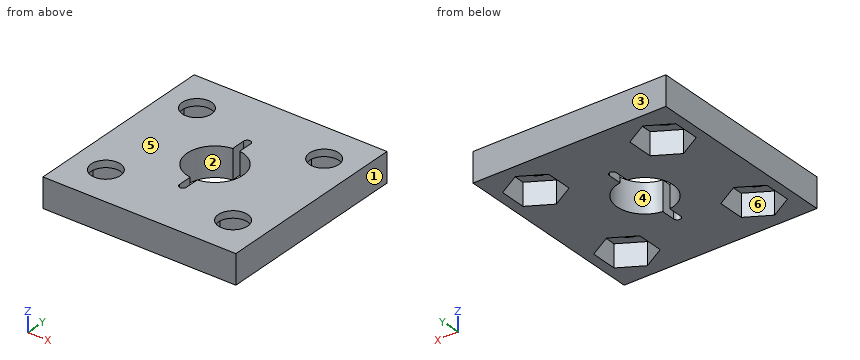
from build123d import *

# Parameters (mm, degrees)
SKETCH1_W           = 35.052
SKETCH1_H           = 35.814
SKETCH1_R           = 2.667
BOSS_EXTRUDE1_DEPTH = 5.334
CUT_EXTRUDE1_DEPTH  = 4.064
SKETCH3_R           = 5.08
CUT_EXTRUDE2_DEPTH  = 6.334
CUT_EXTRUDE3_DEPTH  = 6.334


with BuildPart() as part:
    # Sketch1 → Boss-Extrude1 (new body)
    with BuildSketch(Plane.XY):
        Rectangle(SKETCH1_W, SKETCH1_H)
        with Locations((-11.557, 10.795)):
            Circle(SKETCH1_R, mode=Mode.SUBTRACT)
        with Locations((11.557, 10.795)):
            Circle(SKETCH1_R, mode=Mode.SUBTRACT)
        with Locations((11.557, -10.795)):
            Circle(SKETCH1_R, mode=Mode.SUBTRACT)
        with Locations((-11.557, -10.795)):
            Circle(SKETCH1_R, mode=Mode.SUBTRACT)
    extrude(amount=BOSS_EXTRUDE1_DEPTH)

    # Sketch2 → Cut-Extrude1 (cut)
    with BuildSketch(Plane(origin=(0, 0, 0), x_dir=(-1, 0, 0), z_dir=(0, 0, -1))):
        Polygon((-11.557, 5.955650044), (-7.366, 8.375325022), (-7.366, 13.214674978), (-11.557, 15.634349956), (-15.748, 13.214674978), (-15.748, 8.375325022), align=None)
        Polygon((-11.557, -15.634349956), (-7.366, -13.214674978), (-7.366, -8.375325022), (-11.557, -5.955650044), (-15.748, -8.375325022), (-15.748, -13.214674978), align=None)
        Polygon((11.557, -15.634349956), (15.748, -13.214674978), (15.748, -8.375325022), (11.557, -5.955650044), (7.366, -8.375325022), (7.366, -13.214674978), align=None)
        Polygon((11.557, 5.955650044), (15.748, 8.375325022), (15.748, 13.214674978), (11.557, 15.634349956), (7.366, 13.214674978), (7.366, 8.375325022), align=None)
    extrude(amount=-CUT_EXTRUDE1_DEPTH, mode=Mode.SUBTRACT)

    # Sketch3 → Cut-Extrude2 (cut, through all)
    with BuildSketch(Plane.XY.offset(5.334)):
        Circle(SKETCH3_R)
    extrude(amount=-CUT_EXTRUDE2_DEPTH, mode=Mode.SUBTRACT)

    # Sketch4 → Cut-Extrude3 (cut, through all)
    with BuildSketch(Plane.XY.offset(5.334)):
        with BuildLine():
            Line((-0.635, -7.62), (-0.635, 7.62))
            ThreePointArc((-0.635, 7.62), (0, 8.255), (0.635, 7.62))
            Line((0.635, 7.62), (0.635, -7.62))
            ThreePointArc((0.635, -7.62), (0, -8.255), (-0.635, -7.62))
        make_face()
    extrude(amount=-CUT_EXTRUDE3_DEPTH, mode=Mode.SUBTRACT)


solid = part.part
Read the model definition and answer for the solid it produces. Units are mm, in the model's axes. Face numbers are marked on the shaded views. A direction names the side the tool comes from. Coordinates: 2 decimals unless noted, no trailing zeros. Order: outer loops, then holes, each group sorted by start corner. A loop starts at its lowest first (then second) coordinate and runs counter-clockwise, first axis right, second up. Notation, with made-up numbers: (68, 12.25) -> (81, 12.25) arc R21 ccw to (81, 28.25) -> close; hole circle Ø7 at (-19, -32). An arc over 180 degrees is marked (long way). Answer as a JSON object with one key per item and string values.
1) Consider line 1 along X through (y, z) = (-11, 0.85); line 2 along X through (y, z) = (0, 4.75); line 3 along Y through (x, z) = (-13, 4.2). Determine where each line is inside the solid, lowest interval first. Write a range as from..to.
Model answer:
{"line 1": "x = -17.53..-15.75, -7.37..7.37, 15.75..17.53", "line 2": "x = -17.53..-5.08, 5.08..17.53", "line 3": "y = -17.91..-13.04, -8.55..8.55, 13.04..17.91"}
2) A tool of negligible diameter and unlimited length cuts with its end or side. For the marked faces 4, 5 and 6, from which of +Z, -Z, +X, -X, +Y, -Y can it reach the whole face along a straight path? Write none if from no direction.
Model answer:
{"face 4": "+Z, -Z", "face 5": "+Z, +X, -X, +Y, -Y", "face 6": "-Z"}
3) A cutting plane is placed at D-D, the plane y = 9. Determine the outline of the cut face in (x, z).
Model answer:
{"outline": "(-17.53, 0) -> (-15.75, 0) -> (-15.75, 4.06) -> (-13.53, 4.06) -> (-13.53, 5.33) -> (-17.53, 5.33) -> close; (-9.58, 4.06) -> (-7.37, 4.06) -> (-7.37, 0) -> (7.37, 0) -> (7.37, 4.06) -> (9.58, 4.06) -> (9.58, 5.33) -> (-9.58, 5.33) -> close; (13.53, 4.06) -> (15.75, 4.06) -> (15.75, 0) -> (17.53, 0) -> (17.53, 5.33) -> (13.53, 5.33) -> close"}
4) This flat-tipped pin is pushed along its axis until it touches: pin 1 (7 mm diameter, centred on x = -11.557, y = 10.795, fed in from -Z). Where does it stop, or does it pass through?
Model answer:
{"pin 1": "stops at z = 4.06"}
5) The mould has two halves that part along X. Classify the marked faces 1, 2 and 3: released by +X, released by -X, zero draft, split by the parting line, or undercut.
Model answer:
{"face 1": "released by +X", "face 2": "undercut", "face 3": "zero draft"}
6) A cutting plane is placed at B-B, the plane y = 0.5. Determine the outline of the cut face in (x, z).
Model answer:
{"outline": "(-17.53, 0) -> (-5.06, 0) -> (-5.06, 5.33) -> (-17.53, 5.33) -> close; (5.06, 0) -> (17.53, 0) -> (17.53, 5.33) -> (5.06, 5.33) -> close"}
7) A cutting plane is placed at A-A, the plane x = 0. Determine the outline of the cut face in (y, z) (3 decimals).
Model answer:
{"outline": "(-17.907, 0) -> (-8.255, 0) -> (-8.255, 5.334) -> (-17.907, 5.334) -> close; (8.255, 0) -> (17.907, 0) -> (17.907, 5.334) -> (8.255, 5.334) -> close"}
8) A cutting plane is placed at C-C, the plane x = 9.5. Determine the outline of the cut face in (y, z), plus the area to 3 significant figures.
Model answer:
{"outline": "(-17.91, 0) -> (-14.45, 0) -> (-14.45, 4.06) -> (-12.49, 4.06) -> (-12.49, 5.33) -> (-17.91, 5.33) -> close; (-9.1, 4.06) -> (-7.14, 4.06) -> (-7.14, 0) -> (7.14, 0) -> (7.14, 4.06) -> (9.1, 4.06) -> (9.1, 5.33) -> (-9.1, 5.33) -> close; (12.49, 4.06) -> (14.45, 4.06) -> (14.45, 0) -> (17.91, 0) -> (17.91, 5.33) -> (12.49, 5.33) -> close", "area": "123 mm²"}
